CAD build for the part. Positions are in the model's coordinates, mm. Face numbers are marked on the shaded views. Round coordinates to 2 decimals unless told otherwise and drop trailing zeros. Loops run counter-clockwise (first coordinate to the right, second up) from the corner with the lowest first, then second, coordinate; pieces in that order, holes last.
Autodesk Inventor part; units mm, degrees
ref_plane "YZ Plane" through (0, 0, 0) normal (1, 0, 0) x (0, 1, 0)
ref_plane "XZ Plane" through (0, 0, 0) normal (0, 1, 0) x (-1, 0, 0)
ref_plane "XY Plane" through (0, 0, 0) normal (0, 0, 1) x (1, 0, 0)
sketch "Sketch1" plane through (0, 0, 0) normal (0, 1, 0) x (-1, 0, 0)
  circle A0 centre (0, 0) radius 9.5
  circle A1 centre (0, 0) radius 6.5
  dimension "d0" = 13
  dimension "d1" = 3
extrude "Extrusion1" add sketch "Sketch1" along normal blind 30
sketch "Sketch2" plane through (0, 30, 0) normal (0, 1, 0) x (1, 0, 0)
  circle A0 centre (0, 0) radius 6.5
extrude "Extrusion2" add sketch "Sketch2" against normal blind 7
sketch "Sketch3" plane through (0, 30, 0) normal (0, 1, 0) x (1, 0, 0)
  circle A0 centre (0, 0) radius 2.2
  dimension "d6" = 4.4
extrude "Extrusion3" [suppressed]
sketch "Sketch6" plane through (0, 0, 0) normal (0, 0, 1) x (1, 0, 0)
  circle A0 centre (0, 36) radius 8.75
  line L0 (6.5, 23) -> (-6.5, 23)
  line L1 (9.5, 30) -> (-9.5, 30)
  line L2 (0, 0) -> (0, 49.5814)
  point P0 (0, 27.25)
  point P1 (0, 30)
  point P2 (6.3689, 30)
  point P3 (0, 44.75)
  dimension "d24" = 17.5
  dimension "d25" = 6
  dimension "d26" = 0
revolve "Revolution2" add sketch "Sketch6" angle 360 about axis through (0, 0, 0) along (0, 1, 0) picked at (0.649, 39.7602) contours A0 L1 L2
fillet "Fillet5" radius 3 1 edges at (9.5, 30, 0)
fillet "Fillet6" radius 2 1 edges at (-6.3689, 30, 0)
sketch "Sketch8" plane through (0, 23, 0) normal (0, -1, 0) x (1, 0, 0)
  circle A0 centre (0, 0) radius 5.5
  circle A1 centre (0, 0) radius 6.5
  dimension "d34" = 1
extrude "Extrusion6" add sketch "Sketch8" along normal blind 7
sketch "Sketch7" plane through (0, 0, 0) normal (1, 0, 0) x (0, 1, 0)
  circle A0 centre (20, 0) radius 2.5
  line L0 (27, -9.5) -> (27, 9.5)
  point P0 (0, 0)
  dimension "d30" = 5
  dimension "d31" = 7
extrude "Extrusion5" cut sketch "Sketch7" along normal blind 10
sketch "Sketch4" plane through (0, 0, 0) normal (1, 0, 0) x (0, 1, 0)
  circle A0 centre (38, 0) radius 8.75
  line L0 (30, -9.5) -> (30, 9.5)
  line L1 (12.9825, 0) -> (37.4487, 0)
  point P0 (0, 0)
  point P1 (36.75, 0)
  point P2 (19.25, 0)
  dimension "d9" = 17.5
  dimension "d11" = 8
properties part number "Ballholder"
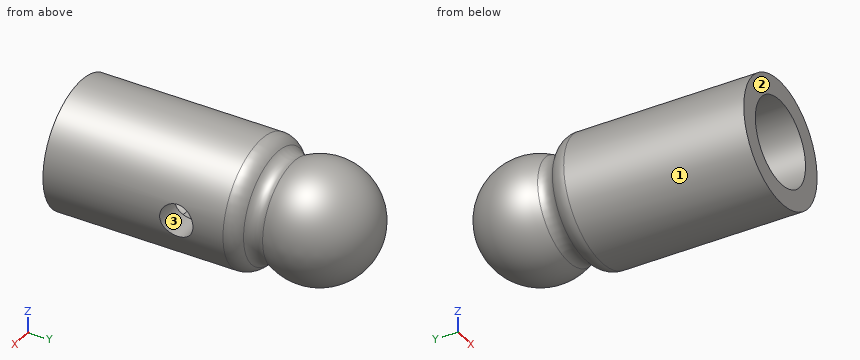
Item 1: Cut at B-B, the plane y = 36. Give the cut face in (x, z).
Answers follow:
outline: circle Ø17.5 at (0, 0)
Item 2: Cut at C-C, the plane x = 0. Give the cut face in (y, z).
Answers follow:
outline: (0, -9.5) - (27, -9.5) arc R3 ccw to (29.39, -8.31) arc R2 cw to (31.92, -7.74) arc R8.75 ccw (long way) to (31.92, 7.74) arc R2 cw to (29.39, 8.31) arc R3 ccw to (27, 9.5) - (0, 9.5) - (0, 6.5) - (16, 6.5) - (16, 5.5) - (23, 5.5) - (23, -5.5) - (16, -5.5) - (16, -6.5) - (0, -6.5) - close
Item 3: Probe line 1 (Z direction, x = 0, y = 12); line 2 (Z direction, x = 4.5, y = 5); line 3 (X direction, y = 6, z = 5). List the from-to ranges inside material, lowest first.
Answers follow:
line 1: z = -9.5 to -6.5, 6.5 to 9.5
line 2: z = -8.37 to -4.69, 4.69 to 8.37
line 3: x = -8.08 to -4.15, 4.15 to 8.08
Item 4: Cut at D-D, the plane y = 20. Give the cut face in (x, z), plus the area to 3 significant figures.
Answers follow:
outline: (4.9, -2.5) arc R5.5 cw (long way) to (4.9, 2.5) - (9.17, 2.5) arc R9.5 ccw (long way) to (9.17, -2.5) - close
area: 168 mm2
Item 5: Two-plate mould, pull along Z, no slides. Class the marked faces 1, 2 and 3: released by +Z, released by -Z, zero draft, split by the parting line, or undercut.
Answers follow:
face 1: split by the parting line
face 2: zero draft
face 3: undercut
Item 6: Flat gauge pins, fed straight in: P1, Ø1.5, axis at y = 33.5, z = 4, coming from the +X side; P2, Ø1, axis at x = -1, z = -4, coming from the -Y side; P3, Ø1.5, axis at x = -4, y = 23.5, coming from the +Z side. Where does each tip first touch, or does it go through?
Answers follow:
P1: stops at x = 7.8
P2: stops at y = 23
P3: stops at z = 8.93
Item 7: Cut at A-A, the plane z = 0. Give the cut face in (x, y).
Answers follow:
outline: (-9.5, 0) - (-6.5, 0) - (-6.5, 16) - (-5.5, 16) - (-5.5, 23) - (5.5, 23) - (5.5, 22.5) - (9.5, 22.5) - (9.5, 27) arc R3 ccw to (8.31, 29.39) arc R2 cw to (7.74, 31.92) arc R8.75 ccw (long way) to (-7.74, 31.92) arc R2 cw to (-8.31, 29.39) arc R3 ccw to (-9.5, 27) - close; (5.5, 16) - (6.5, 16) - (6.5, 0) - (9.5, 0) - (9.5, 17.5) - (5.5, 17.5) - close
